Geometry: see drawing. Coordinates: mm, zero at the bounding-box minimum. Coordinates: 2 decimals unless noted, no trailing zeros. Write each loop counter-clockwise with the first axis right and the second up, starting at its lowest first coordinate (ties: lowest second). Pieces come first, ordered by that corner, then holes. Notation, with made-up numbers: M 21,13 L 72,13 A17 ccw 72,30 Z; hole C 38.25,-33.75 d6. An arc over 180 degrees is marked long. Write item = value, one per line. Start each with the question number.
1. Section query C-C (x = 43). Output: boundary loops of the cut face in (y, z).
2. Section query A-A (y = 13.45). Output: boundary loops of the cut face in (x, z) (3 decimals), then the cut area to 3 significant figures.
3. Line query: line 1 along Y through (x, z) = (16, 31.5); line 2 along X through (y, z) = (13, 26); line 3 along X through (y, z) = (11.5, 40). Output: solid intervals per line, ascending.
4. Section query B-B (z = 8). Output: boundary loops of the cut face in (x, y) (3 decimals).
5. Pin query (flat end, axial travel): pin 1 Ø3 at (x, y) = (15.885, 13.45) entering from -Z. Return the tip coordinate at first contact, or that it passes through.
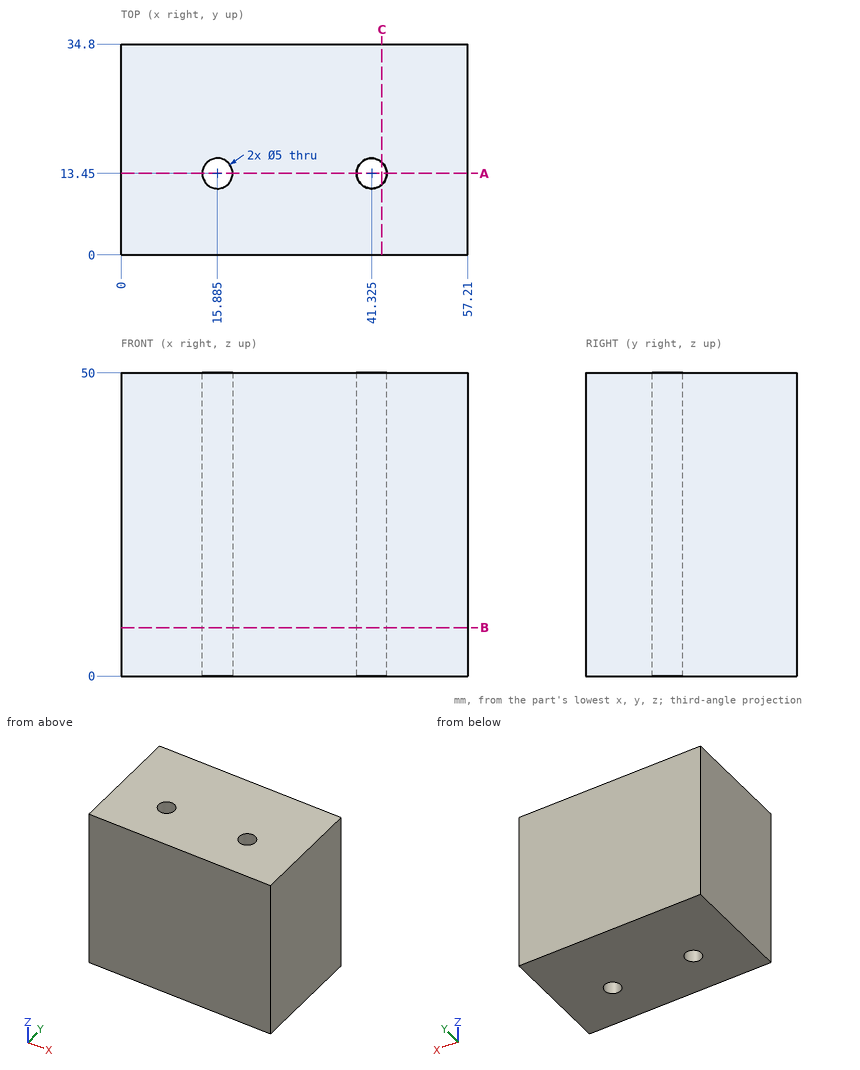
Results are:
q1.outline = M 0,0 L 11.59,0 L 11.59,50 L 0,50 Z; M 15.31,0 L 34.8,0 L 34.8,50 L 15.31,50 Z
q2.outline = M 0,0 L 13.385,0 L 13.385,50 L 0,50 Z; M 18.385,0 L 38.825,0 L 38.825,50 L 18.385,50 Z; M 43.825,0 L 57.21,0 L 57.21,50 L 43.825,50 Z
q2.area = 2,360 mm^2
q3.line_1 = 0 to 10.95, 15.95 to 34.8
q3.line_2 = 0 to 13.43, 18.34 to 38.87, 43.78 to 57.21
q3.line_3 = 0 to 14.32, 17.45 to 39.76, 42.89 to 57.21
q4.outline = M 0,0 L 57.21,0 L 57.21,34.8 L 0,34.8 Z; hole C 15.885,13.45 d5; hole C 41.325,13.45 d5
q5.pin_1 = through
